Input: dimensioned drawing with shaded views. Units: mm. Origin: part minimum x, y, z. Coordinates: 2 decimals unless noted, no trailing zeros. Order: outer loops, then holes, each group sorted by start corner. A loop starts at its lowest first (then second) coordinate and runs counter-clockwise, first axis right, second up. Notation, with made-up numbers: (-11, 80) - (32, 80) arc R5 ccw to (32, 85) - close; hole circle Ø4 at (35.25, 80). An arc over 180 degrees is marked (long way). One line per question, with ' | ' between items. Start each with the question number.
(1) Contact query for flat-ended pins moving along their axis: P1, Ø4.5, axis at x = 55.28, y = 50.7, coming from the +Z side; P2, Ø4, axis at x = 44.45, y = 56.95, coming from the +Z side (1 decimal). Output: stop coordinate, or through.
(2) Section D-D (z = 2.4). Count the separate pieces of the cut face and the enclosed holes in it, then the cut area to 4 significant figures.
(3) Line query: line 1 along Y through (x, z) = (12.7, 2.05); line 2 along Y through (x, z) = (71, 1); line 3 along X through (y, z) = (79, 1). Output: solid intervals per line, ascending.
(4) Section B-B (x = 76.2). Return the cut outline in (y, z) (1 decimal), then the cut area to 3 significant figures.
(5) Section A-A (y = 44.45). Return the cut outline in (x, z) (1 decimal).
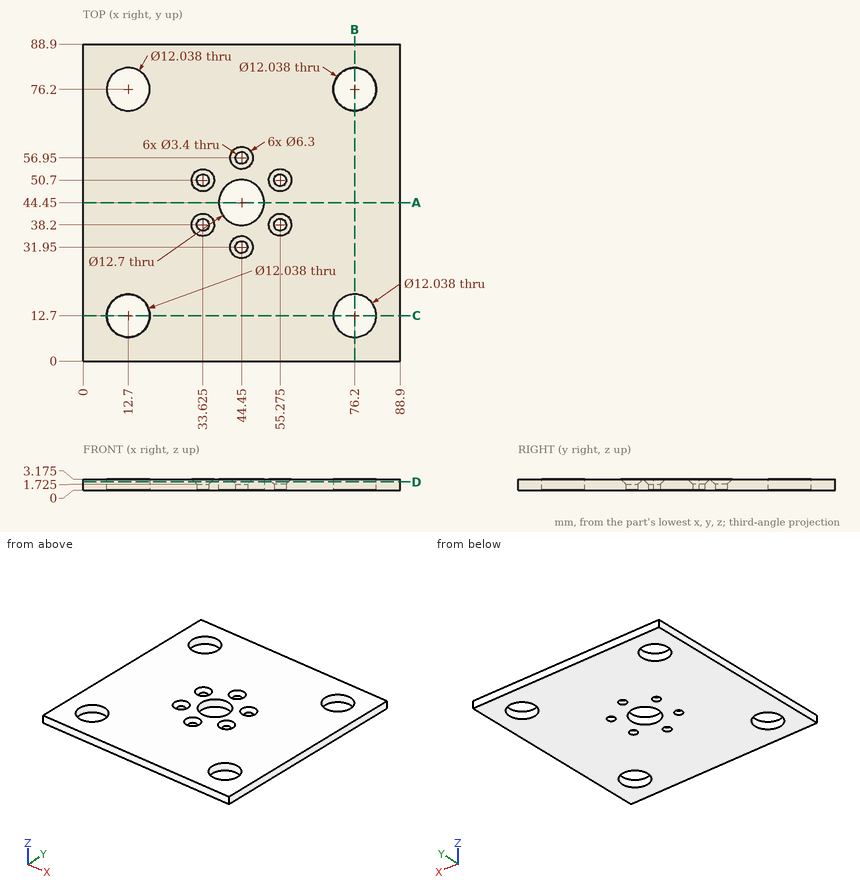
Response values:
1) P1: stops at z = 2.28 | P2: stops at z = 2
2) separate pieces: 1 | enclosed holes: 11 | area: 7,215 mm²
3) line 1: y = 0 to 6.68, 18.72 to 70.18, 82.22 to 88.9 | line 2: y = 0 to 9.67, 15.73 to 73.17, 79.23 to 88.9 | line 3: x = 0 to 7.37, 18.03 to 70.87, 81.53 to 88.9
4) outline: (0, 0) - (6.7, 0) - (6.7, 3.2) - (0, 3.2) - close; (18.7, 0) - (70.2, 0) - (70.2, 3.2) - (18.7, 3.2) - close; (82.2, 0) - (88.9, 0) - (88.9, 3.2) - (82.2, 3.2) - close | area: 206 mm²
5) outline: (0, 0) - (38.1, 0) - (38.1, 3.2) - (0, 3.2) - close; (50.8, 0) - (88.9, 0) - (88.9, 3.2) - (50.8, 3.2) - close
